Answer from the drawing. Dimensions are ordinates in mm from the lowest x, y and z of the part. Coordinates: 2 decimals unless noted, no trailing zeros. Order: outer loops, then holes, each group sorted by start corner. A loop starts at its lowest first (then second) coordinate and runs counter-clockwise, first axis right, second up. Notation, with made-up numbers: (33, -27.5) -> (76, -27.5) arc R16 cw to (76, -1.5) -> close; hole circle Ø10 at (48, 34.5). An arc over 180 degrees is marked (long way). Use CSV: the item, a comma, the result in double quotes.
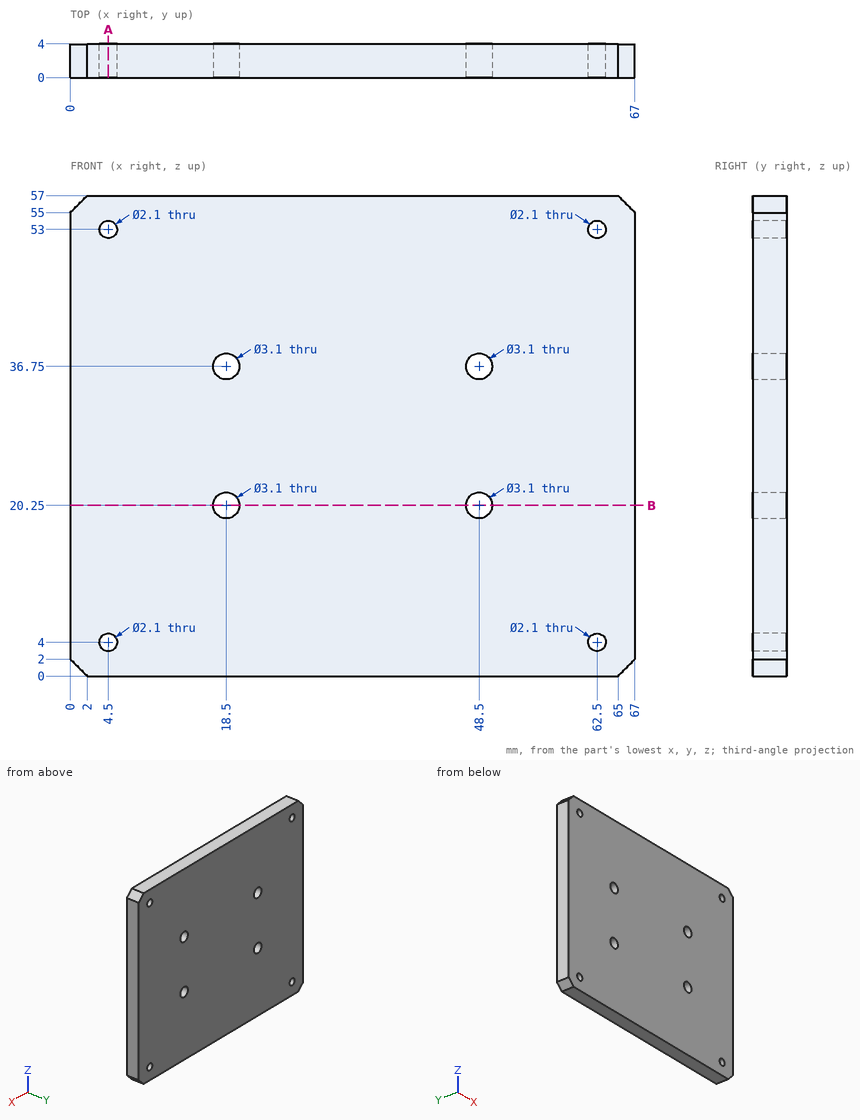
Item 1: Straight lines are drawn through the part: line 1 along X through (y, z) = (1.3, 20.25); line 2 along X through (y, z) = (0.9, 53); line 3 along Z through (x, y) = (48, 3.15). For each, find the intervals that lie inside material, in ascending order.
Return value:
line 1,"x = 0 to 16.95, 20.05 to 46.95, 50.05 to 67"
line 2,"x = 0 to 3.45, 5.55 to 61.45, 63.55 to 67"
line 3,"z = 0 to 18.78, 21.72 to 35.28, 38.22 to 57"
Item 2: Find section A-A, the plane x = 4.5. Give the vertices of the cut face in (y, z), then the cut area to 3 significant figures.
Return value:
outline,"(0, 0) -> (4, 0) -> (4, 2.95) -> (0, 2.95) -> close; (0, 5.05) -> (4, 5.05) -> (4, 51.95) -> (0, 51.95) -> close; (0, 54.05) -> (4, 54.05) -> (4, 57) -> (0, 57) -> close"
area,"211 mm^2"
Item 3: Find section B-B, the plane z = 20.25. Give the vertices of the cut face in (x, y), then the cut area to 3 significant figures.
Return value:
outline,"(0, 0) -> (16.95, 0) -> (16.95, 4) -> (0, 4) -> close; (20.05, 0) -> (46.95, 0) -> (46.95, 4) -> (20.05, 4) -> close; (50.05, 0) -> (67, 0) -> (67, 4) -> (50.05, 4) -> close"
area,"243 mm^2"
